Read the model definition and answer for the solid it produces. Units are mm, in the model's axes. A direction names the side the tool comes from. Coordinates: 2 decimals unless noted, no trailing zeros. Order: outer loops, then holes, each group sorted by start corner. A loop starts at its lowest first (then second) coordinate and runs counter-clockwise, first axis right, second up. Notation, with made-up numbers: M 32.25,69 L 79.25,69 A9 ccw 79.25,75 Z; hole C 73,64.25 d8. An arc over 180 degrees is marked long. One line per question, with ' | ' between items. Start each with the question number.
1) Find section C-C, the plane y = -7. Write down the section's boundary in (x, z), plus the area to 3 significant figures.
2) The mould has two halves that part along Y. Classify faces 3 (the face through (21, -33.7, 0.2)), 4 (the face through (0, -49.1, -9)), 5 (the face through (15.272, -17.235, 2.465)): +Y half, -Y half, draft (parallel to the pull), parting line (faces both ways), or undercut.
3) Find section B-B, the plane y = -15.5. Write down the section's boundary in (x, z).
4) A tool of negligible diameter and unlimited length cuts with its end or side. For faces 1 (the face through (0, -44.1, -12)), 2 (the face through (0, -47, -24)), from which of +Z, -Z, +X, -X, +Y, -Y can it reach the whole face along a straight path? Write none if from no direction.
5) Find section D-D, the plane z = -2.5. Write down the section's boundary in (x, y), plus the area to 3 significant figures.
6) Consider probe 1 along Y at (x, z) = (-15.5, 2.85); probe 2 along Y at (x, z) = (14, -20.25); probe 3 along Z at (x, y) = (12, -18.5). Determine where each line is inside the solid, lowest interval first.
7) Find section A-A, the plane x = -15.5. Write down the section's boundary in (y, z).
8) Given P1, Ø21, axis at x = 6.5, y = -27, coming from the -Z side; P2, Ø1, axis at x = -8, z = -19, coming from the +Y side; P3, Ø3, axis at x = -15.5, y = -15.5, coming from the -Z side, each flat-ended and moving along its own axis, determine where each tip first touches the part or whether it passes through.
Autodesk Inventor part; units mm, degrees
ref_plane "YZ Plane" through (0, 0, 0) normal (1, 0, 0) x (0, 1, 0)
ref_plane "XZ Plane" through (0, 0, 0) normal (0, 1, 0) x (-1, 0, 0)
ref_plane "XY Plane" through (0, 0, 0) normal (0, 0, 1) x (1, 0, 0)
ref_plane "Work Plane1" through (0, 0, 0) normal (0, 0, 1) x (1, 0, 0)
sketch "Sketch1" plane through (0, 0, 0) normal (0, 0, 1) x (1, 0, 0)
  circle A0 centre (0, 0) radius 11
  circle A1 centre (-15.5, -15.5) radius 1.75
  circle A2 centre (15.5, -15.5) radius 1.75
  circle A3 centre (15.5, 15.5) radius 1.75
  circle A4 centre (-15.5, 15.5) radius 1.75
  line L0 (-21, 21) -> (21, 21)
  line L1 (-21, -21) -> (-21, 21)
  line L2 (21, -21) -> (-21, -21)
  line L3 (21, 21) -> (21, -21)
  line L4 (40.7911, -42.1) -> (-34.1821, -42.1)
  line L5 (21, -44.1) -> (-21, -44.1)
  arc A5 (-10.3333, -3.7712) -> (-21, -5.6569) centre (-15.5, -5.6569) ccw
  arc A6 (-10.3333, -3.7712) -> (10.3333, -3.7712) centre (0, 0) ccw
  arc A7 (21, -5.6569) -> (10.3333, -3.7712) centre (15.5, -5.6569) ccw
  line L6 (-21, -5.6569) -> (-21, -44.1)
  line L7 (21, -5.6569) -> (21, -44.1)
  line L8 (-21, -21) -> (21, -21)
  line L9 (21, -21) -> (21, -49.1)
  line L10 (21, -49.1) -> (-21, -49.1)
  line L11 (-21, -49.1) -> (-21, -21)
  point P0 (0, 0)
  dimension "d0" = 2
  dimension "d1" = 5
extrude "Extrusion1" add sketch "Sketch1" along normal blind 5 contours A0 A7 L3 L2 L1 A5 | L2 L7 L4 L6 | L4 L7 L5 L6 | L5 L9 L10 L11
sketch "Sketch2" plane through (0, 0, 0) normal (0, 0, -1) x (-1, 0, 0)
  line L0 (-21, -49.1) -> (21, -49.1)
  line L1 (21, -5.6569) -> (21, -49.1)
  line L2 (-21, -49.1) -> (21, -49.1)
  line L3 (21, -49.1) -> (21, -44.1)
  line L4 (21, -44.1) -> (-21, -44.1)
  line L5 (-21, -44.1) -> (-21, -49.1)
  point P0 (0, 0)
  dimension "d4" = 5
extrude "Extrusion2" add sketch "Sketch2" along normal blind 24
properties part number "Shelf Braket"
Report:
1) outline: M -21,0 L -8.49,0 L -8.49,5 L -21,5 Z; M 8.49,0 L 21,0 L 21,5 L 8.49,5 Z | area: 125 mm^2
2) face 3: draft | face 4: -Y half | face 5: undercut
3) outline: M -21,0 L -17.25,0 L -17.25,5 L -21,5 Z; M -13.75,0 L 13.75,0 L 13.75,5 L -13.75,5 Z; M 17.25,0 L 21,0 L 21,5 L 17.25,5 Z
4) face 1: -Z, +X, -X, +Y | face 2: -Z, +X, -X, +Y, -Y
5) outline: M -21,-49.1 L 21,-49.1 L 21,-44.1 L -21,-44.1 Z | area: 210 mm^2
6) probe 1: y = -49.1 to -17.25, -13.75 to -0.16 | probe 2: y = -49.1 to -44.1 | probe 3: z = 0 to 5
7) outline: M -49.1,-24 L -44.1,-24 L -44.1,0 L -17.25,0 L -17.25,5 L -49.1,5 Z; M -13.75,0 L -0.16,0 L -0.16,5 L -13.75,5 Z
8) P1: stops at z = 0 | P2: stops at y = -44.1 | P3: passes through
